Read the model definition and answer for the solid it produces. Units are mm, in the model's axes. Round coordinates to 2 decimals unless told otherwise and drop trailing zeros. Order: outer loops, then holes, each group sorted by start corner. A loop starts at its lowest first (then second) coordinate and runs counter-clockwise, first axis right, second up. Notation, with made-up numbers: (-24.75, 65.25) - (9.25, 65.25) arc R16 cw to (9.25, 72.25) - close; hole circle Ø4 at (70.25, -20). An arc over 180 degrees is marked (long way). Put each result on its own line as item: value. Start each with the question number.
Q1. Each of these flat-tipped pins is pushed along its axis until it touches: pin 1 Ø6.5 at (x, z) = (6.23, 26) entering from -Y; pin 2 Ø4.5 at (x, z) = (6.23, -26) entering from -Y. Where does it stop, or does it pass through?
Q2. For a pull along X with two mould halves and no side action, classify faces 1 (the face through (18.4, -17.24, 36.93)), 2 (the face through (-19, -17, 0)), 3 (the face through (7.242, -32.188, -27.941)) as pulls with the +X half, pulls with the -X half, needs draft (parallel to the pull), parting line crosses it, or undercut.
Q3. Section A-A on z = 26 is taken. Give the vertices of the cut face in (x, y), then the cut area to 3 significant figures.
Q4. Section B-B on x = -12.5 is taken. Give the vertices of the cut face in (y, z), then the cut area to 3 significant figures.
Q5. Find the intervals of material crossed by line 1 along Z through (x, y) = (-12.5, -10.5); line 2 along Z through (x, y) = (7, -21.5); line 3 along X through (y, z) = (-13.5, 26.5), in increasing order. Write a range as from..to.
from build123d import *

# Parameters (mm, degrees)
F0_W     = 38
F0_H     = 75
F0_R     = 1.25
F0_R_2   = 2
F1_DEPTH = 35
F2_SIZE2 = 3
F2_SIZE  = 3
F3_R     = 2
F4_R     = 1


with BuildPart() as f1:
    # F0 (on Front) → F1 (new body)
    with BuildSketch(Plane.XZ):
        Rectangle(F0_W, F0_H)
        with Locations((-12.5, -26)):
            Circle(F0_R, mode=Mode.SUBTRACT)
        with Locations((6.232371, -26)):
            Circle(F0_R_2, mode=Mode.SUBTRACT)
        with Locations((-12.5, 26)):
            Circle(F0_R, mode=Mode.SUBTRACT)
        with Locations((6.232371, 26)):
            Circle(F0_R_2, mode=Mode.SUBTRACT)
    extrude(amount=F1_DEPTH)

    # F2
    f2_edges = [f1.edges().sort_by_distance(p)[0] for p in [
        (4.232371, -35, 26),
        (4.232371, -35, -26),
    ]]
    chamfer(f2_edges, length=F2_SIZE, length2=F2_SIZE2)

    # F3
    f3_edges = [f1.edges().sort_by_distance(p)[0] for p in [
        (-19, -17.5, 37.5),
        (-19, -17.5, -37.5),
        (19, -17.5, -37.5),
        (19, -17.5, 37.5),
    ]]
    fillet(f3_edges, radius=F3_R)

    # F4
    f4_edges = [f1.edges().sort_by_distance(p)[0] for p in [
        (-19, -35, 0),
    ]]
    fillet(f4_edges, radius=F4_R)


solid = f1.part
Findings:
1. pin 1: y = -33.25
1. pin 2: y = -32.25
2. face 1: pulls with the +X half
2. face 2: pulls with the -X half
2. face 3: undercut
3. outline: (-19, -34) arc R1 ccw to (-18, -35) - (-13.75, -35) - (-13.75, 0) - (-19, 0) - close; (-11.25, -35) - (1.23, -35) - (4.23, -32) - (4.23, 0) - (-11.25, 0) - close; (8.23, -32) - (11.23, -35) - (18, -35) arc R1 ccw to (19, -34) - (19, 0) - (8.23, 0) - close
3. area: 1,090 mm2
4. outline: (-35, -36.5) arc R1 ccw to (-34, -37.5) - (0, -37.5) - (0, -27.25) - (-35, -27.25) - close; (-35, -24.75) - (0, -24.75) - (0, 24.75) - (-35, 24.75) - close; (-35, 27.25) - (0, 27.25) - (0, 37.5) - (-34, 37.5) arc R1 ccw to (-35, 36.5) - close
4. area: 2,450 mm2
5. line 1: -37.5..-27.25, -24.75..24.75, 27.25..37.5
5. line 2: -37.5..-27.85, -24.15..24.15, 27.85..37.5
5. line 3: -19..-13.65, -11.35..4.3, 8.17..19
